Here's how the part is built. I have some questions about the finished solid (model axes, mm). Face numbers are marked on the shaded views. Give positions to 0.01 mm unless a question says otherwise; leave off trailing zeros. Order: outer loops, then holes, each group sorted by start corner. A loop starts at its lowest first (then second) coordinate and runs counter-clockwise, first axis right, second up.
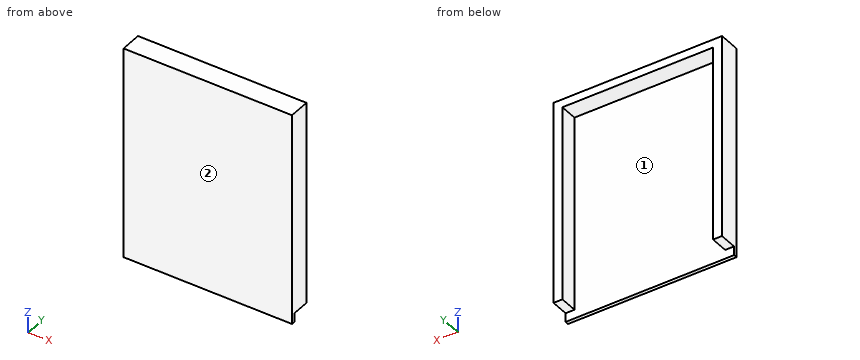
from build123d import *

# Parameters (mm, degrees)
SKETCH1_W           = 241.3
SKETCH1_H           = 304.8
SKETCH1_W_2         = 215.9
SKETCH1_H_2         = 279.4
BOSS_EXTRUDE1_DEPTH = 5.08
BOSS_EXTRUDE2_DEPTH = 25.4


with BuildPart() as part:
    # Sketch1 → Boss-Extrude1 (new body)
    with BuildSketch(Plane(origin=(0, 0, 0), x_dir=(1, 0, 0), z_dir=(0, 1, 0))):
        Rectangle(SKETCH1_W, SKETCH1_H)
        Rectangle(SKETCH1_W_2, SKETCH1_H_2, mode=Mode.SUBTRACT)
        Rectangle(SKETCH1_W_2, SKETCH1_H_2)
    extrude(amount=BOSS_EXTRUDE1_DEPTH)

    # Sketch2 → Boss-Extrude2 (add)
    with BuildSketch(Plane(origin=(0, 5.08, 0), x_dir=(1, 0, 0), z_dir=(0, 1, 0))):
        Polygon((-107.95, 139.7), (-120.65, 139.7), (-120.65, -152.4), (120.65, -152.4), (120.65, 139.7), (107.95, 139.7), (107.95, -140.783695347), (-107.95, -140.783695347), align=None)
    extrude(amount=BOSS_EXTRUDE2_DEPTH)


solid = part.part
Q1. If we section it at A-A on z = 35: List the corners of the cut face in (x, y) for me, plus the area to 3 significant figures.
Filled sheet:
outline: (-120.65, 0) - (120.65, 0) - (120.65, 30.48) - (107.95, 30.48) - (107.95, 5.08) - (-107.95, 5.08) - (-107.95, 30.48) - (-120.65, 30.48) - close
area: 1,870 mm2
Q2. Thinking about a two-plate mould opening in X: for the marked faces 1 and 2, which applies, released by +X, released by -X, zero draft, split by the parting line, or undercut?
Filled sheet:
face 1: undercut
face 2: zero draft
Q3. I'm going to push flat-ended pins straight in: P1, Ø10, axis at x = -69.5, z = -42, coming from the -Y side; P2, Ø1.5, axis at x = 38, z = -32.5, coming from the +Y side; P3, Ø12, axis at x = -55.5, y = 21, coming from the -Z side; P4, Ø14, axis at x = 116, y = 15.5, coming from the -Z side. Where does each tip first touch, or does it pass through?
Filled sheet:
P1: stops at y = 0
P2: stops at y = 5.08
P3: stops at z = 140.78
P4: stops at z = -139.7
Q4. If we section it at C-C on x = -73.5: List the corners of the cut face in (y, z) for me.
Filled sheet:
outline: (0, -152.4) - (5.08, -152.4) - (5.08, 140.78) - (30.48, 140.78) - (30.48, 152.4) - (0, 152.4) - close
Q5. I need wall thicknesses on L1, parallel to X at y = 10.5, z = -38.5; L2, parallel to Y at x = -16, z = 90; L3, parallel to Z at x = 63.5, y = 22.5. Which ranges of each line are inside material? Lowest first, please.
Filled sheet:
L1: x = -120.65 to -107.95, 107.95 to 120.65
L2: y = 0 to 5.08
L3: z = 140.78 to 152.4
Q6. If we section it at B-B on y = 12.5: List the corners of the cut face in (x, z) for me.
Filled sheet:
outline: (-120.65, -139.7) - (-107.95, -139.7) - (-107.95, 140.78) - (107.95, 140.78) - (107.95, -139.7) - (120.65, -139.7) - (120.65, 152.4) - (-120.65, 152.4) - close
